```python
from build123d import *

# Parameters (mm, degrees)
F0_R     = 18.374195
F1_DEPTH = 25.4
F2_R     = 29.366769
F3_DEPTH = 25.4
F4_R     = 5.08
F5_R     = 5.08
F6_SIZE  = 2.54


with BuildPart() as f1:
    # F0 (on Top) → F1 (new body)
    with BuildSketch(Plane.XY):
        Circle(F0_R)
    extrude(amount=-F1_DEPTH)

    # F2 (on Top) → F3 (join)
    with BuildSketch(Plane.XY):
        Circle(F2_R)
    extrude(amount=F3_DEPTH)

    # F4
    f4_edges = [f1.edges().sort_by_distance(p)[0] for p in [
        (-29.366769, 0, 25.4),
    ]]
    fillet(f4_edges, radius=F4_R)

    # F5
    f5_edges = [f1.edges().sort_by_distance(p)[0] for p in [
        (-29.366769, 0, 0),
    ]]
    fillet(f5_edges, radius=F5_R)

    # F6
    f6_edges = [f1.edges().sort_by_distance(p)[0] for p in [
        (-18.374195, 0, -25.4),
    ]]
    chamfer(f6_edges, length=F6_SIZE)


solid = f1.part
```
Source: CAD feature listing. Evaluate the final solid. Frame: model axes, mm. A direction names the side the tool comes from. Coordinates: 2 decimals unless noted, no trailing zeros. Write each loop counter-clockwise with the first axis right and the second up, starting at its lowest first coordinate (ties: lowest second). Pieces come first, ordered by that corner, then holes. Notation, with made-up numbers: (10, 64.5) - (26, 64.5) arc R19 ccw to (26, 96.5) - close; hole circle Ø8 at (48, -4.75). An arc over 180 degrees is marked (long way). Answer as a JSON object with one key per item and string values.
Q1. Set-up query: faces 1 (the flat face through (0, 0, 25.4)), 2 (the cylindrical face through (16.97, -7.04, -11.27)). Return all of +Z, -Z, +X, -X, +Y, -Y with unobstructed straight access to the full face (end or side cutting, diameter ignored); none if empty.
Ans:
{"face 1": "+Z, +X, -X, +Y, -Y", "face 2": "-Z"}
Q2. Material intervals for line 1 (Z direction, x = -14.5, y = -15); line 2 (X direction, y = 0.5, z = -3); line 3 (Y direction, x = 0, z = 12), sorted ascending. Write a range as [from, to].
Ans:
{"line 1": "z = [0, 25.4]", "line 2": "x = [-18.37, 18.37]", "line 3": "y = [-29.37, 29.37]"}
Q3. First-contact query: pin 1 Ø4 at (x, z) = (-19, -5.5) entering from +Y; pin 2 Ø3 at (x, z) = (0.5, 3) entering from +Y; pin 3 Ø3 at (x, z) = (7, 5) entering from +Y. Flat tips, straight axial feed; report the tip coordinate or a pass-through.
Ans:
{"pin 1": "stops at y = 6.97", "pin 2": "stops at y = 29.33", "pin 3": "stops at y = 28.85"}
Q4. Section query A-A, the plane x = 0. Output: boundary loops of the cut face in (y, z), plus the area to 3 significant figures.
Ans:
{"outline": "(-29.37, 5.08) arc R5.08 ccw to (-24.29, 0) - (-18.37, 0) - (-18.37, -22.86) - (-15.83, -25.4) - (15.83, -25.4) - (18.37, -22.86) - (18.37, 0) - (24.29, 0) arc R5.08 ccw to (29.37, 5.08) - (29.37, 20.32) arc R5.08 ccw to (24.29, 25.4) - (-24.29, 25.4) arc R5.08 ccw to (-29.37, 20.32) - close", "area": "2,400 mm2"}
Q5. Section query D-D, the plane z = -3. Output: boundary loops of the cut face in (x, y).
Ans:
{"outline": "circle Ø36.75 at (0, 0)"}
Q6. Section query C-C, the plane z = 15.5. Output: boundary loops of the cut face in (x, y), plus the area to 3 significant figures.
Ans:
{"outline": "circle Ø58.73 at (0, 0)", "area": "2,710 mm2"}
